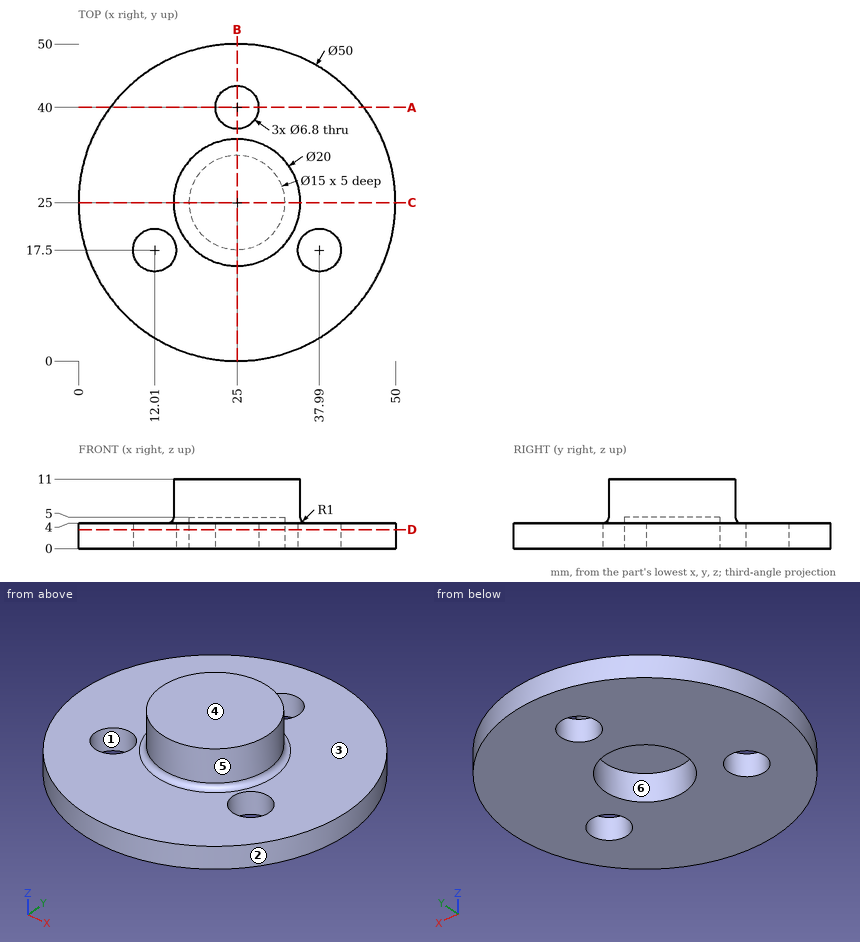
The drawing under review shows one solid part. Ordinate dimensions are in mm from its lowest x, y, z. A direction names the side the tool comes from. Give positions to 0.01 mm unless a question says otherwise; leave off trailing zeros. Write each loop counter-clockwise with the first axis right and the second up, starting at its lowest first coordinate (ties: lowest second). Pieces come first, ordered by that corner, then holes. Notation, with made-up numbers: (59, 68) - (84, 68) arc R29 cw to (84, 93) - close; hole circle Ø3 at (63, 12). An arc over 180 degrees is marked (long way). Answer in a Markdown table with one row per item. Add a question column.
1. Insertion check: P1, Ø5, axis at x = 41.5, y = 40.5, coming from the -Z side; P2, Ø6, axis at y = 34, z = 4.5, coming from the -X side; P3, Ø8, axis at x = 25, y = 40, coming from the +Z side; P4, Ø1.5, axis at x = 27.5, z = 7, coming from the -Y side. Each pin has a flat end and moves straight along its axis. Give the tip position at first contact, or say it passes through.
2. We need section B-B on x = 25. Write out the cut boundary in (y, z).
3. Draft analysis for pull direction X (two halves, no side actions). For the marked faces 1, 2 and 3, state which applies: +X half, -X half, draft (parallel to the pull), parting line (faces both ways), or undercut.
4. We need section D-D on z = 3. Write out the cut boundary in (x, y), then the cut area to 3 significant figures.
5. We need section C-C on y = 25. Write out the cut boundary in (x, z).
6. We need section A-A on y = 40. Write out the cut boundary in (x, z), then the cut area to 3 significant figures.
7. Wall thickness on line 1 along Y through (x, z) = (25, 1.7); line 2 along Z through (x, y) = (39.5, 39); line 3 along Y through (x, z) = (12, 3.25) (1 decimal): over which ranges is each line inside the solid? List them lowest first. Write a range as [from, to].
8. Tool access review of the marked faces 4, 5 and 6: name each direction out of +Z, -Z, +X, -X, +Y, -Y from which nothing blocks a thin tool from reaching the whole face with its end or side.
Ans:
| question | item | result |
|---|---|---|
| 1 | P1 | stops at z = 0 |
| 1 | P2 | stops at x = 0.74 |
| 1 | P3 | stops at z = 4 |
| 1 | P4 | stops at y = 15.15 |
| 2 | outline | (0, 0) - (17.5, 0) - (17.5, 5) - (32.5, 5) - (32.5, 0) - (36.6, 0) - (36.6, 4) - (36, 4) arc R1 cw to (35, 5) - (35, 11) - (15, 11) - (15, 5) arc R1 cw to (14, 4) - (0, 4) - close; (43.4, 0) - (50, 0) - (50, 4) - (43.4, 4) - close |
| 3 | face 1 | undercut |
| 3 | face 2 | parting line |
| 3 | face 3 | draft |
| 4 | outline | circle Ø50 at (25, 25); hole circle Ø6.8 at (12.01, 17.5); hole circle Ø15 at (25, 25); hole circle Ø6.8 at (25, 40); hole circle Ø6.8 at (37.99, 17.5) |
| 4 | area | 1,680 mm^2 |
| 5 | outline | (0, 0) - (17.5, 0) - (17.5, 5) - (32.5, 5) - (32.5, 0) - (50, 0) - (50, 4) - (36, 4) arc R1 cw to (35, 5) - (35, 11) - (15, 11) - (15, 5) arc R1 cw to (14, 4) - (0, 4) - close |
| 6 | outline | (5, 0) - (21.6, 0) - (21.6, 4) - (5, 4) - close; (28.4, 0) - (45, 0) - (45, 4) - (28.4, 4) - close |
| 6 | area | 133 mm^2 |
| 7 | line 1 | y = [0, 17.5], [32.5, 36.6], [43.4, 50] |
| 7 | line 2 | z = [0, 4] |
| 7 | line 3 | y = [3.6, 14.1], [20.9, 46.4] |
| 8 | face 4 | +Z, +X, -X, +Y, -Y |
| 8 | face 5 | +Z |
| 8 | face 6 | -Z |
